Part model, mm, in its own coordinate system. Face numbers are marked on the shaded views. Round coordinates to 2 decimals unless told otherwise and drop trailing zeros. Order: outer loops, then holes, each group sorted by start corner. A loop starts at its lowest first (then second) coordinate and runs counter-clockwise, first axis right, second up. Notation, with made-up numbers: M 62,39.5 L 95,39.5 A30 ccw 95,64.5 Z; hole C 81,29.5 d6. An arc over 180 degrees is marked long. One line per question, with ' | ' between items.
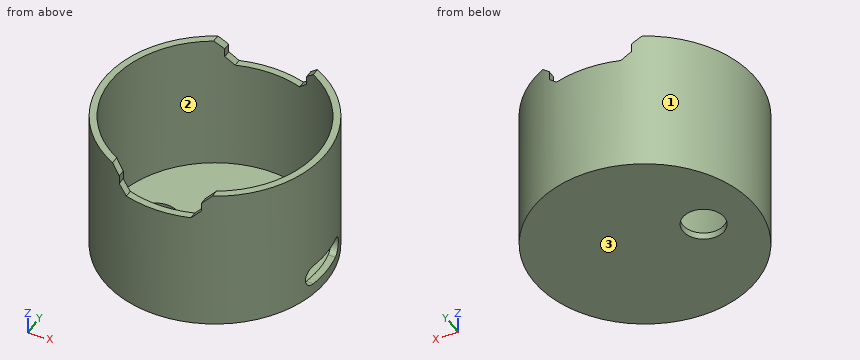
from build123d import *

# Parameters (mm, degrees)
SKETCH010_R     = 19
PAD007_DEPTH    = 25
THICKNESS001_T  = -1.2
BOX001_W        = 14
BOX001_H        = 50
BOX001_DEPTH    = 10
CHAMFER002_SIZE = 1.5
SKETCH012_R     = 3.55
POCKET_DEPTH    = 23
POCKET002_DEPTH = 27


with BuildPart() as part:
    # Sketch010 → Pad007 (new body)
    with BuildSketch(Plane.XY):
        Circle(SKETCH010_R)
    extrude(amount=-PAD007_DEPTH)

    # Thickness001
    thickness001_openings = [part.faces().sort_by_distance(p)[0] for p in [
        (0, 0, 0),
    ]]
    offset(amount=THICKNESS001_T, openings=thickness001_openings)

    # Box001 → Box001 (cut)
    with BuildSketch(Plane(origin=(-7, -24, -4.5), x_dir=(1, 0, 0), z_dir=(0, 0, 1))):
        with Locations((7, 25)):
            Rectangle(BOX001_W, BOX001_H)
    extrude(amount=BOX001_DEPTH, mode=Mode.SUBTRACT)

    # Chamfer002
    chamfer002_edges = [part.edges().sort_by_distance(p)[0] for p in [
        (7, 17.01467, -4.5),
        (7, 17.01467, 0),
        (7, -17.01467, -4.5),
        (7, -17.01467, 0),
        (-7, -17.01467, -4.5),
        (-7, -17.01467, 0),
        (-7, 17.01467, -4.5),
        (-7, 17.01467, 0),
    ]]
    chamfer(chamfer002_edges, length=CHAMFER002_SIZE)

    # Sketch012 → Pocket (cut)
    with BuildSketch(Plane.XY.offset(-4)):
        with Locations((-10, 0)):
            Circle(SKETCH012_R)
    extrude(amount=-POCKET_DEPTH, mode=Mode.SUBTRACT)

    # Sketch013 → Pocket002 (cut)
    with BuildSketch(Plane.YZ.offset(20)):
        with BuildLine():
            ThreePointArc((-3.55, -19.5), (-5.3, -21.25), (-3.55, -23))
            Line((-3.55, -23), (3.55, -23))
            ThreePointArc((3.55, -23), (5.3, -21.25), (3.55, -19.5))
            Line((3.55, -19.5), (-3.55, -19.5))
        make_face()
    extrude(amount=-POCKET002_DEPTH, mode=Mode.SUBTRACT)


with BuildPart() as part_1:
    # Body006 placement: moved
    add(part.part.moved(Location((0, 0, -3))))


solid = part_1.part
1) Saw through at D-D (x = 1). List the corners of the cut face in (y, z), plus the area to 3 significant figures.
The answers:
outline: M -18.97,-28 L 18.97,-28 L 18.97,-7.5 L 17.77,-7.5 L 17.77,-26.8 L -17.77,-26.8 L -17.77,-7.5 L -18.97,-7.5 Z | area: 91.9 mm²
2) Drop flat-ended pins along their axis: pin 1 (1 mm diameter, centred on y = -2, z = -12, fed in from -X); pin 2 (0.6 mm diameter, centred on y = -17, z = -5.5, fed in from +X); pin 3 (1.4 mm diameter, centred on y = -17, z = -5.5, fed in from -X). Give the stop position or say it passes through.
The answers:
pin 1: stops at x = -18.94 | pin 2: stops at x = 9.06 | pin 3: stops at x = -9.76
3) Saw through at A-A (z = -7). List the corners of the cut face in (x, y), plus the area to 3 significant figures.
The answers:
outline: M -6,-18.03 L -6,-16.76 A17.8 cw -6,16.76 L -6,18.03 A19 ccw Z; M 6,-18.03 A19 ccw 6,18.03 L 6,16.76 A17.8 cw 6,-16.76 Z | area: 109 mm²
4) Probe line 1 (Y direction, x = 0, z = -10); line 2 (Z direction, x = 8, y = -14); line 3 (Y direction, x = 11, z = -15). List the from-to ranges inside material, lowest first. Write a range as [from, to].
The answers:
line 1: y = [-19, -17.8], [17.8, 19] | line 2: z = [-28, -26.8] | line 3: y = [-15.49, -13.99], [13.99, 15.49]
5) Saw through at B-B (x = -10). List the corners of the cut face in (y, z).
The answers:
outline: M -16.16,-28 L -3.55,-28 L -3.55,-26.8 L -14.73,-26.8 L -14.73,-3 L -16.16,-3 Z; M 3.55,-28 L 16.16,-28 L 16.16,-3 L 14.73,-3 L 14.73,-26.8 L 3.55,-26.8 Z
6) Saw through at C-C (y = -2.5). List the corners of the cut face in (x, z).
The answers:
outline: M -18.83,-28 L -12.52,-28 L -12.52,-26.8 L -17.62,-26.8 L -17.62,-3 L -18.83,-3 Z; M -7.48,-28 L 18.83,-28 L 18.83,-26 L 17.62,-26 L 17.62,-26.8 L -7.48,-26.8 Z; M 17.62,-22.5 L 18.83,-22.5 L 18.83,-3 L 17.62,-3 Z
7) Two-plate mould, pull along X, no slides. Class the marked faces 1, 2 and 3: released by +X, released by -X, zero draft, split by the parting line, or undercut.
The answers:
face 1: split by the parting line | face 2: undercut | face 3: zero draft
